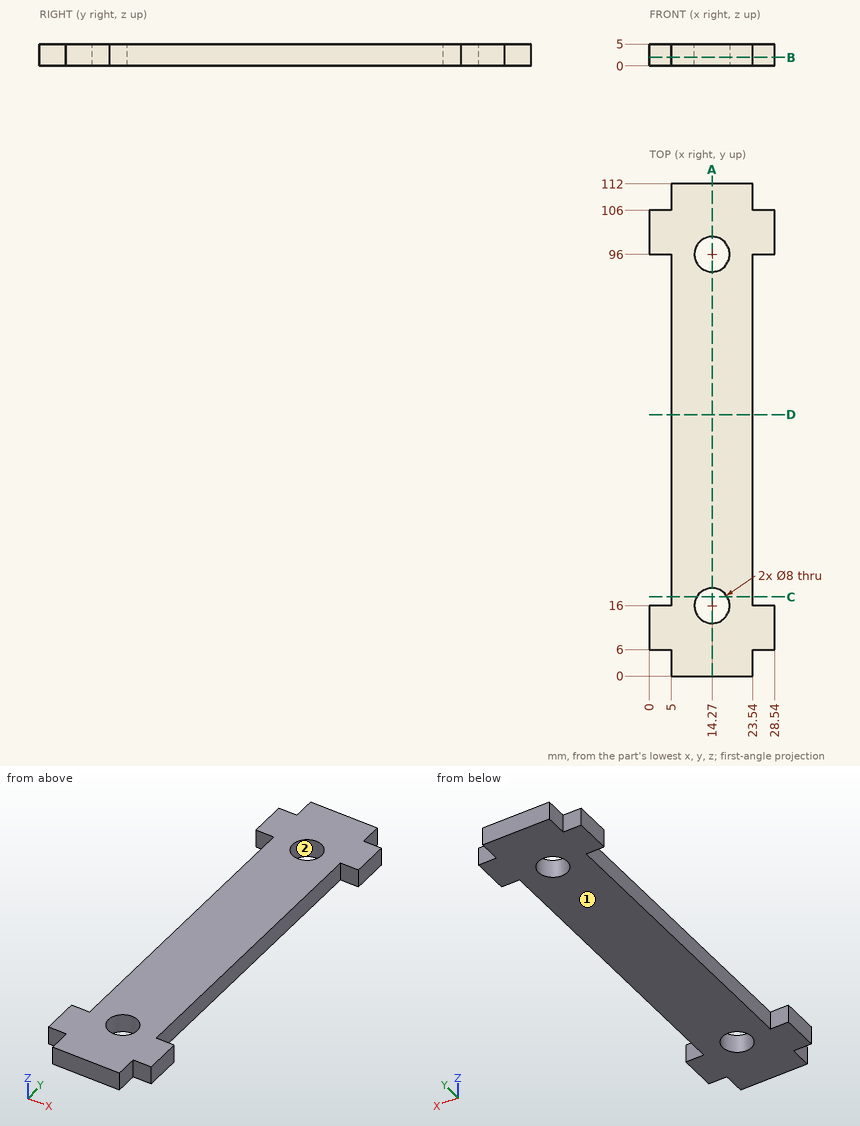
Geometry check sheet. Reference: drawing and pictorial views, mm from the part's lowest x, y, z. Round coordinates to 2 decimals unless told otherwise and drop trailing zeros. Write each loop counter-clockwise with the first axis right and the second up, starting at its lowest first coordinate (ties: lowest second). Pieces come first, ordered by that corner, then holes.
Item 1: Section check A-A (x = 14.27). Record the boundary of the cut face in (y, z).
Determined:
outline: (0, 0) - (12, 0) - (12, 5) - (0, 5) - close; (20, 0) - (92, 0) - (92, 5) - (20, 5) - close; (100, 0) - (112, 0) - (112, 5) - (100, 5) - close
Item 2: Section check B-B (z = 1.95). Record the boundary of the cut face in (x, y).
Determined:
outline: (0, 6) - (5, 6) - (5, 0) - (23.54, 0) - (23.54, 6) - (28.54, 6) - (28.54, 16) - (23.54, 16) - (23.54, 96) - (28.54, 96) - (28.54, 106) - (23.54, 106) - (23.54, 112) - (5, 112) - (5, 106) - (0, 106) - (0, 96) - (5, 96) - (5, 16) - (0, 16) - close; hole circle Ø8 at (14.27, 16); hole circle Ø8 at (14.27, 96)
Item 3: Go/stop test with flat-tipped pins: pin 1 Ø1.5 at (y, z) = (1.5, 3.5) entering from -X; pin 2 Ø2.5 at (x, z) = (26, 2) entering from +Y; pin 3 Ø1.5 at (x, z) = (26, 1.5) entering from -Y; pin 4 Ø1.5 at (x, y) = (3, 60) entering from -Z. Record where each tip stops, or that it passes through.
Determined:
pin 1: stops at x = 5
pin 2: stops at y = 106
pin 3: stops at y = 6
pin 4: passes through
Item 4: Section check C-C (y = 18). Record the boundary of the cut face in (x, z), plus the area to 3 significant figures.
Determined:
outline: (5, 0) - (10.81, 0) - (10.81, 5) - (5, 5) - close; (17.73, 0) - (23.54, 0) - (23.54, 5) - (17.73, 5) - close
area: 58.1 mm2
Item 5: Mould release check, pull along X, two halves, no side actions. Record for the marked faces 1 and 2: +X half, -X half, draft (parallel to the pull), parting line (faces both ways), or undercut.
Determined:
face 1: draft
face 2: undercut
Item 6: Section check D-D (y = 59.5). Record the boundary of the cut face in (x, z), plus the area to 3 significant figures.
Determined:
outline: (5, 0) - (23.54, 0) - (23.54, 5) - (5, 5) - close
area: 92.7 mm2
Item 7: Material ranges on line 1 along Y through (x, z) = (14.27, 3.3); line 2 along Y through (x, z) = (15.5, 3.05); line 3 along X through (y, z) = (30.5, 4.25), recorded low to high.
Determined:
line 1: y = 0 to 12, 20 to 92, 100 to 112
line 2: y = 0 to 12.19, 19.81 to 92.19, 99.81 to 112
line 3: x = 5 to 23.54
